```python
from build123d import *

# Parameters (mm, degrees)
F3_R = 2
F4_R = 2
F6_R = 1


# Not quite as in the source:
# - a fillet or chamfer that OpenCascade refuses, or shapes differently, is made with other operations: its cross-section is extruded or revolved along the edge and cut away or added


with BuildPart() as f1:
    # F0 (on Front) → F1 (revolve)
    with BuildSketch(Plane.XZ):
        with BuildLine():
            ThreePointArc((16.5, 1.2755964417), (11.6628201448, 5.344639677), (10, 11.4430370868))
            Line((10, 11.4430370868), (12, 13.4055894333))
            Line((12, 13.4055894333), (12, 16.5758651609))
            Line((12, 16.5758651609), (9.9997436628, 16.5758651609))
            Line((9.9997436628, 16.5758651609), (9.9997436628, 31.5143950284))
            Line((9.9997436628, 31.5143950284), (7.1613686159, 31.5143950284))
            Line((7.1613686159, 31.5143950284), (7.1613686159, 5.6914240122))
            ThreePointArc((7.1613686159, 5.6914240122), (4.4508587391, 2.967008827), (1, 1.2755964417))
            Line((1, 1.2755964417), (1, 0.0454979338))
            Line((1, 0.0454979338), (16.5, 0))
            Line((16.5, 0), (16.5, 1.2755964417))
        make_face()
    revolve(axis=Axis((0, 0, 19.1986504942), (0, 0, 1)))

    # F2: fillet of radius 5 on 1 edges, made by hand

    # F2_s1 → F2_t2 (revolve, cut)
    with BuildSketch(Plane.XZ):
        with BuildLine():
            ThreePointArc((16.5, 0), (15.750789479, 1.2709297875), (14.6632904097, 2.2678875116))
            ThreePointArc((14.6632904097, 2.2678875116), (15.557168946, 1.7264369439), (16.5, 1.2755964417))
            Line((16.5, 1.2755964417), (16.5, 0))
        make_face()
    revolve(axis=Axis((0, 0, 1.2755964417), (0, 0, 1)), mode=Mode.SUBTRACT)

    # F3
    f3_edges = [f1.edges().sort_by_distance(p)[0] for p in [
        (-12, 0, 13.405589),
    ]]
    fillet(f3_edges, radius=F3_R)

    # F4
    f4_edges = [f1.edges().sort_by_distance(p)[0] for p in [
        (-12, 0, 16.575865),
    ]]
    fillet(f4_edges, radius=F4_R)

    # F5: fillet of radius 3 on 1 edges, made by hand

    # F5_s1 → F5_t2 (revolve, cut)
    with BuildSketch(Plane.XZ):
        with BuildLine():
            ThreePointArc((9.9997436628, 28.5187519631), (9.1774574708, 30.5821381534), (7.1613686159, 31.5143950284))
            Line((7.1613686159, 31.5143950284), (9.9997436628, 31.5143950284))
            Line((9.9997436628, 31.5143950284), (9.9997436628, 28.5187519631))
        make_face()
    revolve(axis=Axis((0, 0, 31.5143950284), (0, 0, 1)), mode=Mode.SUBTRACT)

    # F6
    f6_edges = [f1.edges().sort_by_distance(p)[0] for p in [
        (-7.161369, 0, 31.514395),
    ]]
    fillet(f6_edges, radius=F6_R)


solid = f1.part
```
Could you check a few things on this model? Use its own coordinates, in mm. A direction names the side the tool comes from. Coordinates: 2 decimals unless noted, no trailing zeros. Order: outer loops, then holes, each group sorted by start corner. A loop starts at its lowest first (then second) coordinate and runs counter-clockwise, first axis right, second up. Notation, with made-up numbers: M 17.25,59.25 L 36.25,59.25 A29 ccw 36.25,97.25 Z; hole C 44.5,51 d7. An arc over 180 degrees is marked long. Use a Markdown table: item, result. Add a question column.
Q1. We'd pull the mould along Y, two halves only. Please class faces 1 (the cylindrical face through (-1.302, 9.915, 22.631)), 2 (the conical face through (-1.968, 0.087, 0.043)): pulls with the +Y half, pulls with the -Y half, needs draft (parallel to the pull), parting line crosses it, or undercut.
Q2. Which directions (+Z, -Z, +X, -X, +Y, -Y) give clear straight access to the entire face, cutting with the end or side of a thin tool? Please do faces 3 (the cylindrical face through (11.085, -4.596, 14.413)), 4 (the cylindrical face through (0, -1, 1)).
Q3. If I drill on L1, parallel to Y at x = 0, z = 21.25; L2, parallel to Z at x = 3, y = 1.5; L3, parallel to Y at x = 0, z = 0.45, over which ranges is the centre line in solid material (lowest first)?
Q4. I want a section at A-A on z = 26.5. List the corners of the cut face in (x, y) for me, then the cut area to 3 significant figures.
Q5. I'm going to push flat-ended pins straight in: pin 1 (11.5 mm diameter, centred on x = 0, y = 0, fed in from -Z); pin 2 (3 mm diameter, centred on y = -7, z = 23.5, fed in from +X); pin 3 (6 mm diameter, centred on x = 10, z = 14, fed in from +Y). Where does each tip first touch, or does it pass through?
Checked values:
| question | item | result |
|---|---|---|
| 1 | face 1 | parting line crosses it |
| 1 | face 2 | undercut |
| 2 | face 3 | +Z |
| 2 | face 4 | +Z, -Z |
| 3 | L1 | -10 to -7.16, 7.16 to 10 |
| 3 | L2 | 0.04 to 2.27 |
| 3 | L3 | -16.29 to -1, 1 to 16.29 |
| 4 | outline | C 0,0 d20; hole C 0,0 d14.32 |
| 4 | area | 153 mm² |
| 5 | pin 1 | z = 0.03 |
| 5 | pin 2 | x = 8.35 |
| 5 | pin 3 | y = 9.74 |
